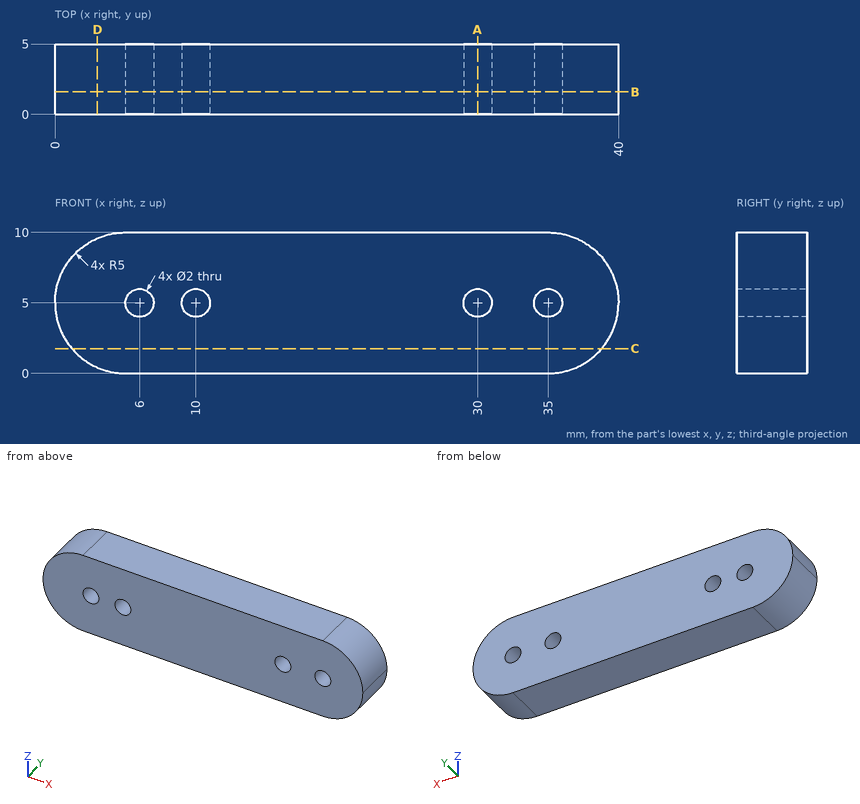
Geometry: see drawing. Coordinates: mm, zero at the bounding-box minimum. Give positions to 0.01 mm unless a question says otherwise; leave off trailing zeros. Loops run counter-clockwise (first coordinate to the right, second up) from the corner with the lowest first, then second, coordinate; pieces in that order, holes last. Notation, with made-up numbers: (-13, 8.5) - (-5, 8.5) arc R11 cw to (-5, 18.5) - close; hole circle Ø11 at (-2, 57). An arc over 180 degrees is marked (long way). Use CSV: the item, a comma, the result in double quotes.
1) Cut plane D-D (x = 3). Output: boundary loops of the cut face in (y, z), and give its area (3 significant figures).
Worked out:
outline,"(0, 0.42) - (5, 0.42) - (5, 9.58) - (0, 9.58) - close"
area,"45.8 mm^2"
2) Line query: line 1 (X direction, y = 3.8, z = 5); line 2 (X direction, y = 0.25, z = 4.5) (1 decimal); line 3 (Z direction, x = 35, y = 1.1). Output: solid intervals per line, ascending.
Worked out:
line 1,"x = 0 to 5, 7 to 9, 11 to 29, 31 to 34, 36 to 40"
line 2,"x = 0 to 5.1, 6.9 to 9.1, 10.9 to 29.1, 30.9 to 34.1, 35.9 to 40"
line 3,"z = 0 to 4, 6 to 10"
3) Cut plane C-C (z = 1.75). Output: boundary loops of the cut face in (x, y).
Worked out:
outline,"(1.2, 0) - (38.8, 0) - (38.8, 5) - (1.2, 5) - close"
4) Pin query (flat end, axial travel): P1, Ø2.5, axis at x = 30, z = 5, coming from the +Y side. Return the tip coordinate at first contact, or that it passes through.
Worked out:
P1,"stops at y = 5"
5) Cut plane A-A (x = 30). Output: boundary loops of the cut face in (y, z).
Worked out:
outline,"(0, 0) - (5, 0) - (5, 4) - (0, 4) - close; (0, 6) - (5, 6) - (5, 10) - (0, 10) - close"
6) Cut plane B-B (y = 1.6). Count the separate pieces of the cut face and the enclosed holes in it, and give its area (3 significant figures).
Worked out:
separate pieces,"1"
enclosed holes,"4"
area,"366 mm^2"
